The drawing under review shows one solid part. Ordinate dimensions are in mm from its lowest x, y, z. A direction names the side the tool comes from. Coordinates: 2 decimals unless noted, no trailing zeros. Write each loop counter-clockwise with the first axis right and the second up, starting at its lowest first coordinate (ties: lowest second). Pieces come first, ordered by that corner, then holes. Notation, with made-up numbers: (52, 9) -> (103, 9) arc R27 cw to (103, 36) -> close; hole circle Ø10 at (77, 70.25). An arc over 180 degrees is marked (long way). One line per item, written item: value. Start each with the question number.
1) For pin 1 Ø10 at (x, z) = (46.5, 12) entering from +Y; pin 2 Ø3 at (y, z) = (31, 35.5) entering from +X, all flat-tipped, find the tip position at first contact; note any pin that passes through.
2) Add section B-B (z = 25). State the section outline as (x, y) points.
3) Add section A-A (x = 45). State the section outline as (y, z) points, and give its area (3 significant figures).
4) For probe 1 along Y at (x, z) = (11, 25); probe 2 along X at (y, z) = (3, 25); probe 3 along Z at (x, y) = (45, 6), list the stretches that pass through material, from the lowest coordinate up. Write a range as from..to.
5) Add section C-C (y = 46). State the section outline as (x, z) points, and give its area (3 significant figures).
6) Mouldability with a two-part tool opening along X and no side actions: class the marked faces 1, 2 and 3 as released by +X, released by -X, zero draft, split by the parting line, or undercut.
7) Add section D-D (x = 17). State the section outline as (y, z) points, and give its area (3 significant figures).
8) Machinability: for the marked faces 4 and 5, which of the approach directions +Z, -Z, +X, -X, +Y, -Y give a long, thin tool a straight path to every point of the face, cutting with its end or side? Answer none if there is none.
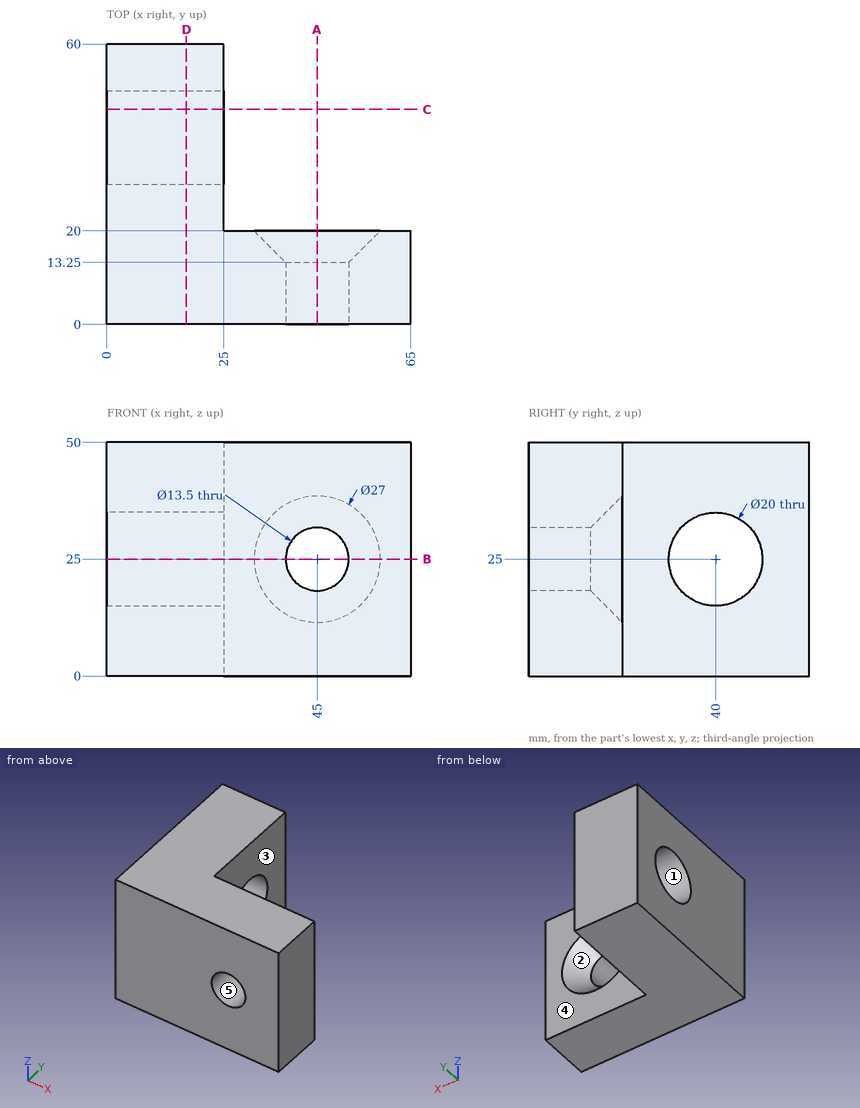
Numbers:
1. pin 1: y = 20
1. pin 2: x = 25
2. outline: (0, 0) -> (38.25, 0) -> (38.25, 13.25) -> (31.5, 20) -> (25, 20) -> (25, 30) -> (0, 30) -> close; (0, 50) -> (25, 50) -> (25, 60) -> (0, 60) -> close; (51.75, 0) -> (65, 0) -> (65, 20) -> (58.5, 20) -> (51.75, 13.25) -> close
3. outline: (0, 0) -> (20, 0) -> (20, 11.5) -> (13.25, 18.25) -> (0, 18.25) -> close; (0, 31.75) -> (13.25, 31.75) -> (20, 38.5) -> (20, 50) -> (0, 50) -> close
3. area: 684 mm²
4. probe 1: 0..30, 50..60
4. probe 2: 0..38.25, 51.75..65
4. probe 3: 0..18.25, 31.75..50
5. outline: (0, 0) -> (25, 0) -> (25, 17) -> (0, 17) -> close; (0, 33) -> (25, 33) -> (25, 50) -> (0, 50) -> close
5. area: 850 mm²
6. face 1: zero draft
6. face 2: undercut
6. face 3: released by +X
7. outline: (0, 0) -> (60, 0) -> (60, 50) -> (0, 50) -> close; hole circle Ø20 at (40, 25)
7. area: 2,690 mm²
8. face 4: +Z, -Z, +X, +Y
8. face 5: +Y, -Y
